from build123d import *

# Parameters (mm, degrees)
F0_W     = 33.3248
F0_H     = 66.650534
F1_DEPTH = 25.4
F2_W     = 17.029665
F2_H     = 50.208108
F2_W_2   = 15.855189
F3_DEPTH = 63.5
F4_R     = 19.855384
F4_R_2   = 10.242902
F5_DEPTH = 50.8


with BuildPart() as f1:
    # F0 (on Front) → F1 (new body)
    with BuildSketch(Plane.XZ):
        with Locations((-77.588384, -2.495724)):
            Rectangle(F0_W, F0_H)
        with Locations((-110.913184, -2.495724)):
            Rectangle(F0_W, F0_H)
    extrude(amount=F1_DEPTH)

    # F2 (on Front) → F3 (join)
    with BuildSketch(Plane.XZ):
        with Locations((-118.91045, -1.027652)):
            Rectangle(F2_W, F2_H)
        with Locations((-68.995954, -1.027652)):
            Rectangle(F2_W_2, F2_H)
    extrude(amount=-F3_DEPTH)

    # F4 (on Front) → F5 (join)
    with BuildSketch(Plane.XZ):
        with Locations((-95.127657, 0)):
            Circle(F4_R)
        with Locations((-95.127657, 0)):
            Circle(F4_R_2, mode=Mode.SUBTRACT)
    extrude(amount=F5_DEPTH)


solid = f1.part
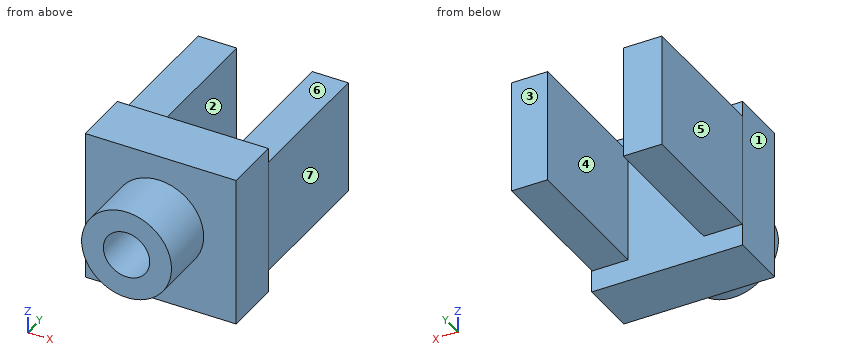
Verification items for the finished model (mm, model axes). Face numbers are marked on the shaded views. A direction names the side the tool comes from. Give positions to 0.01 mm unless a question says otherwise; leave off trailing zeros. Write each loop counter-clockwise with the first axis right and the second up, starting at its lowest first coordinate (ties: lowest second). Pieces come first, ordered by that corner, then holes. Notation, with made-up numbers: M 69.25,-3 L 102.25,-3 A10 cw 102.25,16 Z; hole C 89.25,89.25 d7. An arc over 180 degrees is marked long. Put each result on its own line as item: value. Start each with the question number.
1. Section check D-D (y = -36.5). Record the cut outline in (x, z).
2. Draft check along X on the marked faces 1, 2 and 3. Enter one of: +X half, -X half, draft (parallel to the pull), parting line (faces both ways), or undercut.
3. Go/stop test with flat-tipped pins: pin 1 Ø5 at (x, y) = (-69, 44) entering from -Z; pin 2 Ø6 at (y, z) = (49.5, -24) entering from +X; pin 3 Ø1.5 at (y, z) = (-33.5, 6) entering from +X. Record where each tip stops, or that it passes through.
4. Scan lines: line 1 along X through (y, z) = (-44.25, 0); line 2 along X through (y, z) = (54, 18.5); line 3 along Y through (x, z) = (-101.5, 9.5). Record each from-to range of solid material in increasing order. Write a range as [from, to].
5. Set-up check for the marked faces 4, 5, 6 and 7: record each of +Z, -Z, +X, -X, +Y, -Y from which the full face is reachable in a straight line by a thin tool's end or side.
6. Section check A-A (y = 21). Record the cut outline in (x, z), and give its area (3 significant figures).
7. Section check B-B (x = -71). Record the cut outline in (y, z).
8. Section check C-C (z = 0). Record the cut outline in (x, y), and give its area (3 significant figures).
Answer list:
1. outline: C -95.13,0 d39.71; hole C -95.13,0 d20.49
2. face 1: -X half
2. face 2: undercut
2. face 3: draft
3. pin 1: z = -26.13
3. pin 2: x = -61.07
3. pin 3: x = -75.98
4. line 1: [-114.98, -105.37], [-84.88, -75.27]
4. line 2: [-127.43, -110.4], [-76.92, -61.07]
4. line 3: [-50.8, 0]
5. face 4: +Z, -Z, +Y
5. face 5: +Z, -Z, -X, +Y
5. face 6: +Z, +X, -X, +Y
5. face 7: +Z, -Z, +X, +Y
6. outline: M -127.43,-26.13 L -110.4,-26.13 L -110.4,24.08 L -127.43,24.08 Z; M -76.92,-26.13 L -61.07,-26.13 L -61.07,24.08 L -76.92,24.08 Z
6. area: 1,650 mm2
7. outline: M -25.4,-35.82 L 0,-35.82 L 0,-26.13 L 63.5,-26.13 L 63.5,24.08 L 0,24.08 L 0,30.83 L -25.4,30.83 Z
8. outline: M -127.58,-25.4 L -114.98,-25.4 L -114.98,-50.8 L -105.37,-50.8 L -105.37,-25.4 L -84.88,-25.4 L -84.88,-50.8 L -75.27,-50.8 L -75.27,-25.4 L -60.93,-25.4 L -60.93,0 L -61.07,0 L -61.07,63.5 L -76.92,63.5 L -76.92,0 L -110.4,0 L -110.4,63.5 L -127.43,63.5 L -127.43,0 L -127.58,0 Z
8. area: 4,270 mm2
